Work out the finished part from the listing and answer in its coordinate system (mm). Face numbers are marked on the shaded views. A direction names the side the tool comes from. Coordinates: 2 decimals unless noted, no trailing zeros. Loops run counter-clockwise (first coordinate to the right, second up) from the corner with the lowest first, then second, coordinate; pieces in that order, holes last. Notation, with made-up numbers: M 24.25,63 L 63.25,63 A10 cw 63.25,81 Z; hole C 42.5,34.5 d9. An arc over 180 degrees is marked long. Write each question's results on one line, items separated by ' | '.
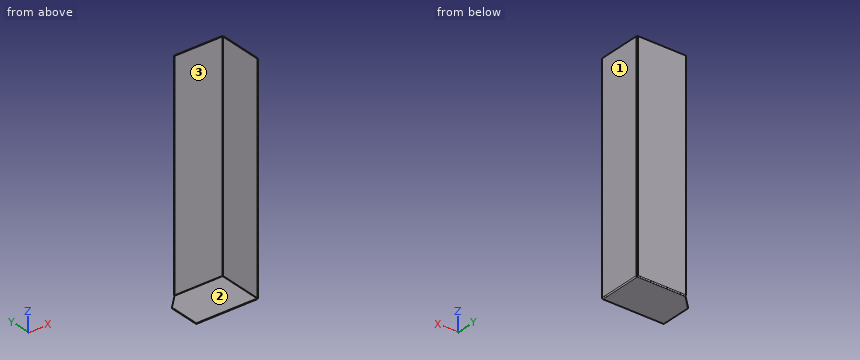
```python
from build123d import *

# Parameters (mm, degrees)
TABAN_FLAN_2_DEPTH            = 1.5
KENAR_FLAN_2_STRIP_W          = 7.4732
KENAR_FLAN_2_STRIP_H          = 1.5
KENAR_FLAN_2_STRIP_CUT_DEPTH  = 110
KENAR_FLAN_2_RELIEF_W         = 8.2232
KENAR_FLAN_2_RELIEF_H         = 0.75
KENAR_FLAN_2_RELIEF_CUT_DEPTH = 1.5
KENAR_FLAN_2_DEPTH            = 110
KENAR_FLAN_4_STRIP_W          = 7.4732
KENAR_FLAN_4_STRIP_H          = 1.5
KENAR_FLAN_4_STRIP_CUT_DEPTH  = 99.2634
KENAR_FLAN_4_DEPTH            = 99.2634


# Sheet-metal steps are written as plain solids
with BuildPart() as part:
    # Çizim1 → Taban-Flanş2 (new body)
    with BuildSketch(Plane.XY):
        Polygon((0, 0), (0, 70), (30, 100), (140, 100), (140, 0), align=None)
    extrude(amount=-TABAN_FLAN_2_DEPTH)

    # Kenar-Flanş2 strip (across the edge) → Kenar-Flanş2 strip cut (cut)
    with BuildSketch(Plane(origin=(140, 100, 0), x_dir=(0, -1, 0), z_dir=(-1, 0, 0))):
        with Locations((-3, -0.75)):
            Rectangle(KENAR_FLAN_2_STRIP_W, KENAR_FLAN_2_STRIP_H)
    extrude(amount=KENAR_FLAN_2_STRIP_CUT_DEPTH, mode=Mode.SUBTRACT)

    # Kenar-Flanş2 relief (on the sheet) → Kenar-Flanş2 relief cut (cut)
    with BuildSketch(Plane(origin=(140, 99.2634, 0), x_dir=(0, -1, 0), z_dir=(0, 0, 1))):
        with Locations((-3.3616, -110.375)):
            Rectangle(KENAR_FLAN_2_RELIEF_W, KENAR_FLAN_2_RELIEF_H)
    extrude(amount=-KENAR_FLAN_2_RELIEF_CUT_DEPTH, mode=Mode.SUBTRACT)

    # Kenar-Flanş2 section (across the edge) → Kenar-Flanş2 (add)
    with BuildSketch(Plane(origin=(140, 100, 0), x_dir=(0, -1, 0), z_dir=(-1, 0, 0))):
        with BuildLine():
            Line((-1.5, 0.7366), (-1.5, 500))
            Line((-1.5, 500), (0, 500))
            Line((0, 500), (0, 0.7366))
            ThreePointArc((0, 0.7366), (0.215745145, 0.215745145), (0.7366, 0))
            Line((0.7366, 0), (0.7366, -1.5))
            ThreePointArc((0.7366, -1.5), (-0.844915027, -0.844915027), (-1.5, 0.7366))
        make_face()
    extrude(amount=KENAR_FLAN_2_DEPTH)

    # Kenar-Flanş4 strip (across the edge) → Kenar-Flanş4 strip cut (cut)
    with BuildSketch(Plane(origin=(140, 0, 0), x_dir=(-1, 0, 0), z_dir=(0, 1, 0))):
        with Locations((-3, -0.75)):
            Rectangle(KENAR_FLAN_4_STRIP_W, KENAR_FLAN_4_STRIP_H)
    extrude(amount=KENAR_FLAN_4_STRIP_CUT_DEPTH, mode=Mode.SUBTRACT)

    # Kenar-Flanş4 section (across the edge) → Kenar-Flanş4 (add)
    with BuildSketch(Plane(origin=(140, 0, 0), x_dir=(-1, 0, 0), z_dir=(0, 1, 0))):
        with BuildLine():
            Line((-1.5, 0.7366), (-1.5, 500))
            Line((-1.5, 500), (0, 500))
            Line((0, 500), (0, 0.7366))
            ThreePointArc((0, 0.7366), (0.215745145, 0.215745145), (0.7366, 0))
            Line((0.7366, 0), (0.7366, -1.5))
            ThreePointArc((0.7366, -1.5), (-0.844915027, -0.844915027), (-1.5, 0.7366))
        make_face()
    extrude(amount=KENAR_FLAN_4_DEPTH)


solid = part.part
```
1) Straight lines are drawn through the part: probe 1 along X at (y, z) = (41.5, 74); probe 2 along Z at (x, y) = (28, 89); probe 3 along Y at (x, z) = (103, 211). For each, find the intervals that lie inside material, in ascending order. Write a range as [from, to].
Check result:
probe 1: [140, 141.5] | probe 2: [-1.5, 0] | probe 3: [100, 101.5]
2) Find section D-D, the plane x = 11.5. Give the vertices of the cut face in (y, z).
Check result:
outline: M 0,-1.5 L 81.5,-1.5 L 81.5,0 L 0,0 Z
3) Which of the six approach directions +Z, -Z, +X, -X, +Y, -Y give full straight-line access (tool end or side, diameter ignored) to the marked faces 1, 2 and 3?
Check result:
face 1: +Z, -Z, +X, +Y, -Y | face 2: +Z, -X, -Y | face 3: +Z, +X, -X, -Y
4) Find section C-C, the plane y = 49.5. Give the vertices of the cut face in (x, z), and give its area (3 significant figures).
Check result:
outline: M 0,-1.5 L 139.26,-1.5 A2.24 ccw 141.5,0.74 L 141.5,500 L 140,500 L 140,0.74 A0.74 cw 139.26,0 L 0,0 Z | area: 961 mm^2
5) Find section B-B, the plane x = 59. Give the vertices of the cut face in (y, z).
Check result:
outline: M 0,-1.5 L 99.26,-1.5 A2.24 ccw 101.5,0.74 L 101.5,500 L 100,500 L 100,0.74 A0.74 cw 99.26,0 L 0,0 Z
6) Given pin 1 Ø12 at (x, z) = (75, 151.5) entering from -Y; pin 2 Ø2 at (y, z) = (43, 231) entering from -X; pin 3 Ø0.7 at (x, z) = (140.5, 183.5) entering from +Y, each flat-ended and moving along its own axis, determine where each tip first touches the part or whether it passes through.
Check result:
pin 1: y = 100 | pin 2: x = 140 | pin 3: y = 99.26
7) Find section A-A, the plane z = 340. Give the vertices of the cut face in (x, y).
Check result:
outline: M 30,100 L 140,100 L 140,101.5 L 30,101.5 Z; M 140,0 L 141.5,0 L 141.5,99.26 L 140,99.26 Z
